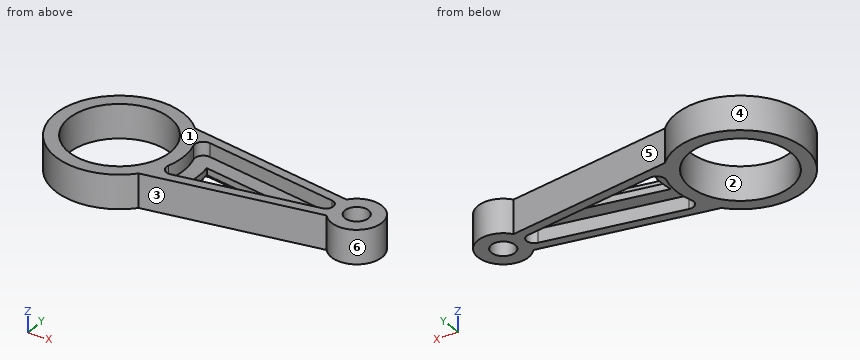
```python
from build123d import *

# Parameters (mm, degrees)
SKETCH1_R           = 30
SKETCH1_R_2         = 7
BOSS_EXTRUDE1_DEPTH = 10
CUT_EXTRUDE1_DEPTH  = 8
CUT_EXTRUDE2_DEPTH  = 161.040619844


with BuildPart() as part:
    # Sketch1 → Boss-Extrude1 (new, symmetric)
    with BuildSketch(Plane.XY):
        with BuildLine():
            Line((27.935473676, 25.760615491), (128.063755469, 9.084385863))
            ThreePointArc((128.063755469, 9.084385863), (155, 0), (128.063755469, -9.084385863))
            Line((128.063755469, -9.084385863), (27.935473676, -25.760615491))
            ThreePointArc((27.935473676, -25.760615491), (-38, 0), (27.935473676, 25.760615491))
        make_face()
        Circle(SKETCH1_R, mode=Mode.SUBTRACT)
        with Locations((140, 0)):
            Circle(SKETCH1_R_2, mode=Mode.SUBTRACT)
    extrude(amount=BOSS_EXTRUDE1_DEPTH, both=True)

    # Sketch2 → Cut-Extrude1 (cut)
    with BuildSketch(Plane.XY.offset(10)):
        with BuildLine():
            Line((41.828554558, 17.870982725), (122.478416149, 4.438857582))
            ThreePointArc((122.478416149, 4.438857582), (126.239130435, 0), (122.478416149, -4.438857582))
            Line((122.478416149, -4.438857582), (41.828554558, -17.870982725))
            ThreePointArc((41.828554558, -17.870982725), (37.231968897, -16.217361812), (36.238855523, -11.43439331))
            ThreePointArc((36.238855523, -11.43439331), (38, 0), (36.238855523, 11.43439331))
            ThreePointArc((36.238855523, 11.43439331), (37.231968897, 16.217361812), (41.828554558, 17.870982725))
        make_face()
    cut_extrude1 = extrude(amount=-CUT_EXTRUDE1_DEPTH, mode=Mode.SUBTRACT)

    # Mirror1: Cut-Extrude1 across plane
    add(cut_extrude1.mirror(Plane.XY), mode=Mode.SUBTRACT)

    # Sketch3 → Cut-Extrude2 (cut, through all)
    with BuildSketch(Plane.XY.offset(2)):
        with BuildLine():
            ThreePointArc((46.314154572, -7.999942891), (47, 0), (46.314154572, 7.999942891))
            Line((46.314154572, 7.999942891), (94.347826087, 0))
            Line((94.347826087, 0), (46.314154572, -7.999942891))
        make_face()
    extrude(amount=-CUT_EXTRUDE2_DEPTH, mode=Mode.SUBTRACT)


solid = part.part
```
CAD build for the part. Positions are in the model's coordinates, mm. Face numbers are marked on the shaded views. A direction names the side the tool comes from. Round coordinates to 2 decimals unless told otherwise and drop trailing zeros. Write each loop counter-clockwise with the first axis right and the second up, starting at its lowest first coordinate (ties: lowest second). Pieces come first, ordered by that corner, then holes. Notation, with made-up numbers: (-35.75, 75) - (-10.75, 75) arc R27 ccw to (-10.75, 104) - close; hole circle Ø11 at (-16.75, 10.25). An arc over 180 degrees is marked (long way). Write item = value, one per line. Start each with the question number.
Q1. Mould opens along Y. For the marked faces 1, 2, 3 and 4 say: pulls with the +Y half, pulls with the -Y half, needs draft (parallel to the pull), parting line crosses it, or undercut.
Q2. Band-saw the part on C-C (y = -24). Give the cut face in (x, z), then the cut area to 3 significant figures.
Q3. Band-saw the part on A-A (x = 0). Give the cut face in (y, z).
Q4. Band-saw the part on B-B (z = 0). Give the cut face in (x, y), then the cut area to 3 significant figures.
Q5. Drop flat-ended pins along their axis: pin 1 (8 mm diameter, centred on x = -3.5, z = 8, fed in from -Y); pin 2 (18 mm diameter, centred on x = 86, y = 2.5, fed in from +Z); pin 3 (4 mm diameter, centred on y = -6, z = 0.5, fed in from -X); pin 4 (2 mm diameter, centred on y = -24.5, z = 1, fed in from -X). Give the stop position or say it passes through.
Q6. Which spindle directions (+Z, -Z, +X, -X, +Y, -Y) get a long thin tool onto all of the face, cutting with end or side? Do the marked faces 5 and 6. Say none if no direction does.
Q7. Probe L1, parallel to X at y = -3, z = -6.5; L2, parallel to Y at x = 140, z = 4.5; L3, parallel to X at y = 4, z = 4.5. List the from-to ranges inside material, lowest first. Write a range as from..to.
Q8. Band-saw the part on D-D (x = 109). Give the cut face in (y, z), then the cut area to 4 significant figures.
Answers below:
q1.face_1 = needs draft
q1.face_2 = undercut
q1.face_3 = pulls with the -Y half
q1.face_4 = parting line crosses it
q2.outline = (-29.46, -10) - (-18, -10) - (-18, 10) - (-29.46, 10) - close; (18, -10) - (38.51, -10) - (38.51, 10) - (18, 10) - close
q2.area = 639 mm2
q3.outline = (-38, -10) - (-30, -10) - (-30, 10) - (-38, 10) - close; (30, -10) - (38, -10) - (38, 10) - (30, 10) - close
q4.outline = (27.94, -25.76) - (128.06, -9.08) arc R15 ccw (long way) to (128.06, 9.08) - (27.94, 25.76) arc R38 ccw (long way) to start; hole circle Ø60 at (0, 0); hole (46.31, -8) - (94.35, 0) - (46.31, 8) arc R47 cw to start; hole circle Ø14 at (140, 0)
q4.area = 4,980 mm2
q5.pin_1 = -38
q5.pin_2 = 10
q5.pin_3 = -37.79
q5.pin_4 = -29.86
q6.face_5 = +Z, -Z, +Y
q6.face_6 = +Z, -Z
q7.L1 = -37.88..-29.85, 29.85..37.88, 125.09..133.68, 146.32..154.7
q7.L2 = -15..-7, 7..15
q7.L3 = -37.79..-29.73, 29.73..37.79, 123.8..134.26, 145.74..154.46
q8.outline = (-12.26, -10) - (-6.68, -10) - (-6.68, -2) - (6.68, -2) - (6.68, -10) - (12.26, -10) - (12.26, 10) - (6.68, 10) - (6.68, 2) - (-6.68, 2) - (-6.68, 10) - (-12.26, 10) - close
q8.area = 276.5 mm2
